```python
from build123d import *

# Parameters (mm, degrees)
SKETCH1_R           = 1.6
BOSS_EXTRUDE1_DEPTH = 4


with BuildPart() as part:
    # Sketch1 → Boss-Extrude1 (new body)
    with BuildSketch(Plane.XY):
        with BuildLine():
            Line((-81.241225793, -6.924028443), (-42.192224122, -15.594407241))
            add(Edge.make_bspline(
                [(-42.192224122, -15.594407241), (-29.042309964, -18.51419346), (-20.671199627, -4), (3, -4)],
                knots=[0, 0, 0, 0, 1, 1, 1, 1], degree=3))
            ThreePointArc((3, -4), (7, 0), (3, 4))
            add(Edge.make_bspline(
                [(-40.458148362, -7.784606907), (-35.521822822, -8.880660851), (-24.58512885, 4), (3, 4)],
                knots=[0, 0, 0, 0, 1, 1, 1, 1], degree=3))
            Line((-40.458148362, -7.784606907), (-79.507150033, 0.885771891))
            ThreePointArc((-79.507150033, 0.885771891), (-84.27908808, -2.152090396), (-81.241225793, -6.924028443))
        make_face()
        with Locations((-22.192224122, -4.956209462)):
            Circle(SKETCH1_R, mode=Mode.SUBTRACT)
        Circle(SKETCH1_R, mode=Mode.SUBTRACT)
    extrude(amount=BOSS_EXTRUDE1_DEPTH)


solid = part.part
```
Verification items for the finished model (mm, model axes). A direction names the side the tool comes from. Coordinates: 2 decimals unless noted, no trailing zeros. Loops run counter-clockwise (first coordinate to the right, second up) from the corner with the lowest first, then second, coordinate; pieces in that order, holes last. Notation, with made-up numbers: (87, 42.25) -> (106, 42.25) arc R21 ccw to (106, 62.25) -> close; hole circle Ø1 at (6, 49.5). An arc over 180 degrees is marked (long way). Answer in a Markdown table with one row per item.
1) Access from +Z, -Z, +X, -X, +Y, -Y to the whole of each face (thin tool, end or side, straight path). Record for faces 1 (the face through (-59.71, -3.51, 1.97)), 2 (the face through (-1.27, -0.97, 1.97)).
The answers:
| item | result |
|---|---|
| face 1 | +Z, -Z, +Y |
| face 2 | +Z, -Z |
2) Scan lines: line 1 along Y through (x, z) = (0, 2.45); line 2 along Y through (x, z) = (-23, 1.3); line 3 along Y through (x, z) = (-18, 0.65). Record each from-to range of solid material in increasing order. Write a range as from..to.
The answers:
| item | result |
|---|---|
| line 1 | y = -4.08..-1.6, 1.6..3.95 |
| line 2 | y = -10.63..-6.34, -3.58..-0.54 |
| line 3 | y = -8.34..1.14 |
3) Section check A-A (z = 1.55). Give the number of separate pieces and of enclosed holes in the cut face, and give its area (3 significant figures).
The answers:
| item | result |
|---|---|
| separate pieces | 1 |
| enclosed holes | 2 |
| area | 757 mm2 |
4) Depth check by flat-ended pin: P1, Ø1.5, axis at x = -7, z = 3.5, coming from the +Y side; P2, Ø1, axis at y = -11.5, z = 3.5, coming from the +X side; P3, Ø3.5, axis at x = 0, y = 0, coming from the -Z side; P4, Ø2, axis at y = -6, z = 2, coming from the -X side. Enter the tip coordinate at first touch or a pass-through.
The answers:
| item | result |
|---|---|
| P1 | stops at y = 3.49 |
| P2 | stops at x = -23.76 |
| P3 | stops at z = 0 |
| P4 | stops at x = -83.85 |
5) Draft check along X on faces 3 (the face through (-20.666, -4.476, 1.972)), 4 (the face through (7, 0, 2)), 5 (the face through (-39, -10, 0)). Enter one of: released by +X, released by -X, zero draft, split by the parting line, or undercut.
The answers:
| item | result |
|---|---|
| face 3 | undercut |
| face 4 | released by +X |
| face 5 | zero draft |
6) Section check C-C (x = -43). Record the cut outline in (y, z).
The answers:
| item | result |
|---|---|
| outline | (-15.42, 0) -> (-7.22, 0) -> (-7.22, 4) -> (-15.42, 4) -> close |
